from build123d import *

# Parameters (mm, degrees)
SKIZZE1_W                       = 75
SKIZZE1_H                       = 65
AUFSATZ_LINEAR_AUSTRAGEN1_DEPTH = 70
SKIZZE4_W                       = 54.15
SKIZZE4_H                       = 53.3
SCHNITT_LINEAR_AUSTRAGEN1_DEPTH = 73
SKIZZE9_W                       = 3
SKIZZE9_H                       = 1
AUFSATZ_LINEAR_AUSTRAGEN2_DEPTH = 73
SCHNITT_LINEAR_AUSTRAGEN3_REACH = 117.974
SKIZZE12_W                      = 7.812260402
SKIZZE12_H                      = 53.3
SCHNITT_LINEAR_AUSTRAGEN4_REACH = 123.45
SKIZZE15_W                      = 12.3
SKIZZE15_H                      = 22.6


# Read off the part's stored shape, not the designer's step: Ø3.0 (3) Durchmesser Bohrung1, Ø3.0 (3) Durchmesser Bohrung2
with BuildPart() as part:
    # Skizze1 → Aufsatz-Linear austragen1 (new body)
    with BuildSketch(Plane.XY):
        with Locations((37.5, 32.5)):
            Rectangle(SKIZZE1_W, SKIZZE1_H)
    extrude(amount=AUFSATZ_LINEAR_AUSTRAGEN1_DEPTH)

    # Skizze4 → Schnitt-Linear austragen1 (cut)
    with BuildSketch(Plane.ZY):
        with Locations((32.925, 32.5)):
            Rectangle(SKIZZE4_W, SKIZZE4_H)
    extrude(amount=-SCHNITT_LINEAR_AUSTRAGEN1_DEPTH, mode=Mode.SUBTRACT)

    # Skizze9 → Aufsatz-Linear austragen2 (add)
    with BuildSketch(Plane.ZY):
        with Locations((12.35, 58.65)):
            Rectangle(SKIZZE9_W, SKIZZE9_H)
        with Locations((12.35, 6.35)):
            Rectangle(SKIZZE9_W, SKIZZE9_H)
    extrude(amount=-AUFSATZ_LINEAR_AUSTRAGEN2_DEPTH)

    # Skizze12 → Schnitt-Linear austragen3 (cut, up to next)
    with BuildSketch(Plane(origin=(0, 0, 60), x_dir=(-1, 0, 0), z_dir=(0, 0, -1)), mode=Mode.PRIVATE) as schnitt_linear_austragen3_sk1:
        with Locations((-3.906130201, 32.5)):
            Rectangle(SKIZZE12_W, SKIZZE12_H)
    schnitt_linear_austragen3_tool1 = extrude(schnitt_linear_austragen3_sk1.sketch, amount=-SCHNITT_LINEAR_AUSTRAGEN3_REACH, mode=Mode.PRIVATE) & part.part
    add(schnitt_linear_austragen3_tool1.solids().sort_by_distance((3.90613, 32.5, 60))[0], mode=Mode.SUBTRACT)

    # Ø3.0 (3) Durchmesser Bohrung1 outline → Ø3.0 (3) Durchmesser Bohrung1 (revolve, cut)
    with BuildSketch(Plane(origin=(50.669703956, 18.6, 0), x_dir=(1, 0, 0), z_dir=(0, -1, 0))):
        Polygon((0, 70), (0, 61.098709071), (1.5, 62), (1.5, 70), align=None)
    revolve(axis=Axis((50.669703956, 18.6, 0), (0, 0, 1)), mode=Mode.SUBTRACT)

    # 3.0 _3_ Durchmesser Bohrung1 2 outline → 3.0 _3_ Durchmesser Bohrung1 2 (revolve, cut)
    with BuildSketch(Plane(origin=(50.669703956, 46.4, 0), x_dir=(1, 0, 0), z_dir=(0, -1, 0))):
        Polygon((0, 70), (0, 61.098709071), (1.5, 62), (1.5, 70), align=None)
    revolve(axis=Axis((50.669703956, 46.4, 0), (0, 0, 1)), mode=Mode.SUBTRACT)

    # Skizze15 → Schnitt-Linear austragen4 (cut, up to next)
    with BuildSketch(Plane.XY.offset(70), mode=Mode.PRIVATE) as schnitt_linear_austragen4_sk1:
        with Locations((51.013730389, 32.5)):
            Rectangle(SKIZZE15_W, SKIZZE15_H)
    schnitt_linear_austragen4_tool1 = extrude(schnitt_linear_austragen4_sk1.sketch, amount=-SCHNITT_LINEAR_AUSTRAGEN4_REACH, mode=Mode.PRIVATE) & part.part
    add(schnitt_linear_austragen4_tool1.solids().sort_by_distance((51.01373, 32.5, 70))[0], mode=Mode.SUBTRACT)

    # Ø3.0 (3) Durchmesser Bohrung2 outline → Ø3.0 (3) Durchmesser Bohrung2 (revolve, cut)
    with BuildSketch(Plane(origin=(0, 62.075, 2.925), x_dir=(0, 1, 0), z_dir=(0, 0, -1))):
        Polygon((1.5, 8), (0, 8.901290929), (0, 0), (1.5, 0), align=None)
    revolve(axis=Axis((0, 62.075, 2.925), (1, 0, 0)), mode=Mode.SUBTRACT)

    # 3.0 _3_ Durchmesser Bohrung2 2 outline → 3.0 _3_ Durchmesser Bohrung2 2 (revolve, cut)
    with BuildSketch(Plane(origin=(0, 2.925, 2.925), x_dir=(0, 1, 0), z_dir=(0, 0, -1))):
        Polygon((1.5, 8), (0, 8.901290929), (0, 0), (1.5, 0), align=None)
    revolve(axis=Axis((0, 2.925, 2.925), (1, 0, 0)), mode=Mode.SUBTRACT)

    # 3.0 _3_ Durchmesser Bohrung2 3 outline → 3.0 _3_ Durchmesser Bohrung2 3 (revolve, cut)
    with BuildSketch(Plane(origin=(0, 2.925, 67.075), x_dir=(0, 1, 0), z_dir=(0, 0, -1))):
        Polygon((1.5, 8), (0, 8.901290929), (0, 0), (1.5, 0), align=None)
    revolve(axis=Axis((0, 2.925, 67.075), (1, 0, 0)), mode=Mode.SUBTRACT)

    # 3.0 _3_ Durchmesser Bohrung2 4 outline → 3.0 _3_ Durchmesser Bohrung2 4 (revolve, cut)
    with BuildSketch(Plane(origin=(0, 62.075, 67.075), x_dir=(0, 1, 0), z_dir=(0, 0, -1))):
        Polygon((1.5, 8), (0, 8.901290929), (0, 0), (1.5, 0), align=None)
    revolve(axis=Axis((0, 62.075, 67.075), (1, 0, 0)), mode=Mode.SUBTRACT)


solid = part.part
Could you check a few things on this model? Use its own coordinates, in mm. A direction names the side the tool comes from. Coordinates: 2 decimals unless noted, no trailing zeros. Write each loop counter-clockwise with the first axis right and the second up, starting at its lowest first coordinate (ties: lowest second). Pieces come first, ordered by that corner, then holes. Notation, with made-up numbers: (48, 13) - (80, 13) arc R23 ccw to (80, 33) - close; hole circle Ø4 at (70, 17.5). An arc over 180 degrees is marked (long way). Put each result on its own line as item: value. Start each with the question number.
Q1. I'm going to push flat-ended pins straight in: P1, Ø3, axis at y = 49.5, z = 28.5, coming from the -X side; P2, Ø11, axis at y = 36.5, z = 66, coming from the -X side; P3, Ø1, axis at x = 57.5, z = 22, coming from the -Y side; P4, Ø1.8, axis at y = 2.925, z = 67.075, coming from the -X side. Where does each tip first touch, or does it pass through?
Q2. Thinking about a two-plate mould opening in Y: for faces 4 (the flat face through (37, 0, 35)), 5 (the cylindrical face through (4.06, 2.6, 1.46)), 6 (the flat face through (37, 33, 0)), which applies, pulls with the +Y half, pulls with the -Y half, needs draft (parallel to the pull), parting line crosses it, or undercut?
Q3. I want a section at C-C on z = 41.5. Write out the boundary of the cut face in (x, y), plus the area to 3 significant figures.
Q4. Which directions (+Z, -Z, +X, -X, +Y, -Y) give clear straight access to the entire face, cutting with the end or side of a thin tool? Please do faces 1 (the flat face through (51, 43.8, 65)), 2 (the flat face through (0, 28, 4)), 3 (the flat face through (36, 5.85, 8)).
Q5. I want a section at A-A on x = 22. Write out the boundary of the cut face in (y, z), plus the area to 3 significant figures.
Q6. I want a section at B-B on y = 35. Write out the boundary of the cut face in (x, z), plus the area to 3 significant figures.
Q7. Please list where these lines run through material, in increasing order: L1, parallel to Z at x = 9, y = 58.5; L2, parallel to Y at x = 14.5, z = 51; L3, parallel to Y at x = 29.5, z = 13.
Checks:
1. P1: x = 73
1. P2: x = 7.81
1. P3: y = 0
1. P4: x = 8.36
2. face 4: pulls with the -Y half
2. face 5: undercut
2. face 6: needs draft
3. outline: (0, 0) - (75, 0) - (75, 65) - (0, 65) - (0, 59.15) - (73, 59.15) - (73, 5.85) - (0, 5.85) - close
3. area: 984 mm²
4. face 1: +Z
4. face 2: +Z, -Z, -X, +Y, -Y
4. face 3: -X
5. outline: (0, 0) - (65, 0) - (65, 70) - (0, 70) - close; hole (5.85, 5.85) - (59.15, 5.85) - (59.15, 10.85) - (58.15, 10.85) - (58.15, 13.85) - (59.15, 13.85) - (59.15, 60) - (5.85, 60) - (5.85, 13.85) - (6.85, 13.85) - (6.85, 10.85) - (5.85, 10.85) - close
5. area: 1,670 mm²
6. outline: (0, 0) - (75, 0) - (75, 70) - (57.16, 70) - (57.16, 60) - (73, 60) - (73, 5.85) - (0, 5.85) - close; (7.81, 60) - (44.86, 60) - (44.86, 70) - (7.81, 70) - close
6. area: 1,100 mm²
7. L1: 0 to 5.85, 10.85 to 13.85, 60 to 70
7. L2: 0 to 5.85, 59.15 to 65
7. L3: 0 to 6.85, 58.15 to 65
